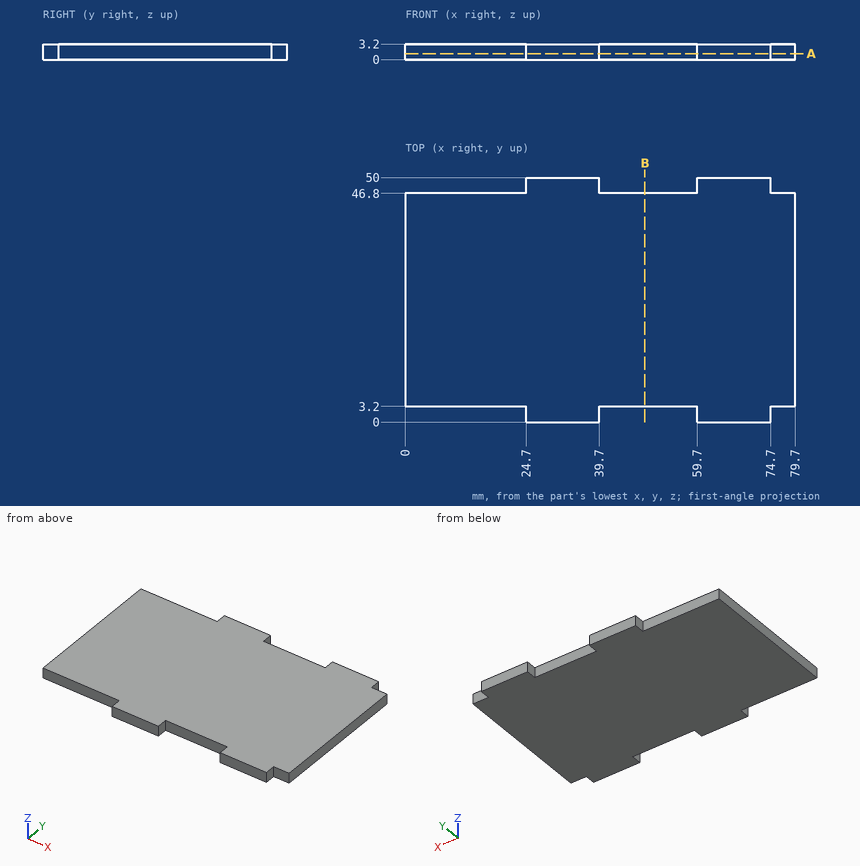
Answer from the drawing. Dimensions are ordinates in mm from the lowest x, y and z of the part. Give positions to 0.01 mm unless a question says otherwise; leave off trailing zeros. Write each loop counter-clockwise with the first axis right and the second up, starting at its lowest first coordinate (ties: lowest second). Pieces come first, ordered by that corner, then holes. Notation, with made-up numbers: (87.5, 9.5) -> (144.5, 9.5) arc R17 ccw to (144.5, 33.5) -> close; hole circle Ø9 at (71, 35). An arc over 180 degrees is marked (long way). One line per question, with ' | ' between items. Start each with the question number.
1. Section B-B (x = 49) is taken. Determine the outline of the cut face in (y, z).
2. Given pin 1 Ø1 at (x, z) = (77, 1) entering from +Y; pin 2 Ø1 at (y, z) = (2.5, 1) entering from -X; pin 3 Ø1.6 at (x, z) = (48, 1) entering from -Y; pin 4 Ø1 at (x, z) = (24.5, 1) entering from -Y, each flat-ended and moving along its own axis, determine where each tip first touches the part or whether it passes through.
3. Find the intervals of material crossed by probe 1 along Y at (x, z) = (48, 2.1), in increasing order.
4. Section A-A (z = 1.25) is taken. Determine the outline of the cut face in (x, y), plus the area to 3 significant figures.
Response values:
1) outline: (3.2, 0) -> (46.8, 0) -> (46.8, 3.2) -> (3.2, 3.2) -> close
2) pin 1: y = 46.8 | pin 2: x = 24.7 | pin 3: y = 3.2 | pin 4: y = 0
3) probe 1: 3.2 to 46.8
4) outline: (0, 3.2) -> (24.7, 3.2) -> (24.7, 0) -> (39.7, 0) -> (39.7, 3.2) -> (59.7, 3.2) -> (59.7, 0) -> (74.7, 0) -> (74.7, 3.2) -> (79.7, 3.2) -> (79.7, 46.8) -> (74.7, 46.8) -> (74.7, 50) -> (59.7, 50) -> (59.7, 46.8) -> (39.7, 46.8) -> (39.7, 50) -> (24.7, 50) -> (24.7, 46.8) -> (0, 46.8) -> close | area: 3,670 mm2
